Autodesk Inventor part; units mm, degrees
ref_plane "YZ Plane" through (0, 0, 0) normal (1, 0, 0) x (0, 1, 0)
ref_plane "XZ Plane" through (0, 0, 0) normal (0, 1, 0) x (-1, 0, 0)
ref_plane "XY Plane" through (0, 0, 0) normal (0, 0, 1) x (1, 0, 0)
ref_plane "Work Plane1" through (0, 0, 0) normal (0, 0, 1) x (1, 0, 0)
sketch "Sketch1" plane through (0, 0, 0) normal (0, 0, 1) x (1, 0, 0)
  line L0 (0, 75.8) -> (40.7, 75.8)
  line L1 (40.7, 65.2) -> (40.7, 75.8) construction
  line L2 (40.7, 65.2) -> (0, 65.2)
  line L3 (0, 65.2) -> (0, 75.8)
  line L4 (0, 0) -> (0, 65.2) construction
  line L5 (40.7, 0) -> (0, 0)
  line L6 (40.7, 0) -> (40.7, 65.2) construction
  line L7 (0, 65.2) -> (40.7, 65.2)
  line L8 (0, -10.6) -> (40.7, -10.6)
  line L9 (0, 0) -> (0, -10.6)
  line L10 (40.7, -10.6) -> (40.7, 0) construction
  line L11 (40.7, 32.6) -> (0, 32.6) construction
  line L12 (0, 32.6) -> (-300, 32.6) construction
  line L13 (30, 75.8) -> (30, 85.8)
  line L14 (-300, 125.8) -> (-300, 32.6)
  line L15 (-300, -60.6) -> (-300, 32.6)
  line L16 (30, 0) -> (30, 65.2)
  line L17 (-3, 85.8) -> (-3, 95.8)
  line L18 (30, 85.8) -> (-3, 85.8)
  line L19 (-3, 95.8) -> (-300, 125.8)
  line L20 (30, -10.6) -> (30, -20.6)
  line L21 (-3, -20.6) -> (-3, -30.6)
  line L22 (30, -20.6) -> (-3, -20.6)
  line L23 (-3, -30.6) -> (-300, -60.6)
  line L24 (-300, 110.2667) -> (-303, 110.2667)
  line L25 (-303, 110.2667) -> (-303, 79.2)
  line L26 (-303, 79.2) -> (-300, 79.2)
  line L27 (-300, 48.1333) -> (-303, 48.1333)
  line L28 (-303, 48.1333) -> (-303, 32.6)
  line L29 (-303, 32.6) -> (-300, 32.6) construction
  line L30 (-303, 79.2) -> (-303, 48.1333) construction
  line L31 (-303, 110.2667) -> (-303, 125.8) construction
  line L32 (-303, 125.8) -> (-300, 125.8) construction
  line L33 (-301.5, 110.2667) -> (-301.5, 94.7333) construction
  line L34 (-301.5, 94.7333) -> (-303, 94.7333) construction
  line L35 (-300, -45.0667) -> (-303, -45.0667)
  line L36 (-303, -45.0667) -> (-303, -14)
  line L37 (-303, -14) -> (-300, -14)
  line L38 (-300, 17.0667) -> (-303, 17.0667)
  line L39 (-303, 17.0667) -> (-303, 32.6)
  line L40 (-3, 75.8) -> (-3, 85.8)
  dimension "d0" = 300
  dimension "d1" = 10
  dimension "d2" = 50
  dimension "d3" = 30
  dimension "d6" = 10
  dimension "d10" = 3
extrude "Extrusion1" add sketch "Sketch1" along normal blind 3
sketch "Sketch3" plane through (0, 0, 3) normal (0, 0, 1) x (1, 0, 0)
  line L0 (0, 75.8) -> (30, 75.8)
  line L1 (30, 75.8) -> (30, 85.8)
  line L2 (30, 85.8) -> (-3, 85.8)
  line L3 (-3, 85.8) -> (-3, 95.8)
  line L4 (-3, 95.8) -> (-300, 125.8)
  line L5 (-300, 125.8) -> (-300, 110.2667)
  line L6 (-300, 110.2667) -> (-303, 110.2667)
  line L7 (-303, 110.2667) -> (-303, 79.2)
  line L8 (-303, 79.2) -> (-300, 79.2)
  line L9 (-300, 79.2) -> (-300, 48.1333)
  line L10 (-300, 48.1333) -> (-303, 48.1333)
  line L11 (-303, 48.1333) -> (-303, 17.0667)
  line L12 (-303, 17.0667) -> (-300, 17.0667)
  line L13 (-300, 17.0667) -> (-300, -14)
  line L14 (-300, -14) -> (-303, -14)
  line L15 (-303, -14) -> (-303, -45.0667)
  line L16 (-303, -45.0667) -> (-300, -45.0667)
  line L17 (-300, -45.0667) -> (-300, -60.6)
  line L18 (-300, -60.6) -> (-3, -30.6)
  line L19 (-3, -30.6) -> (-3, -20.6)
  line L20 (-3, -20.6) -> (30, -20.6)
  line L21 (30, -20.6) -> (30, -10.6)
  line L22 (30, -10.6) -> (0, -10.6)
  line L23 (0, -10.6) -> (0, 0)
  line L24 (0, 0) -> (30, 0)
  line L25 (30, 0) -> (30, 65.2)
  line L26 (30, 65.2) -> (0, 65.2)
  line L27 (0, 65.2) -> (0, 75.8)
properties part number "Stand 1" material "Wood (Oak)"
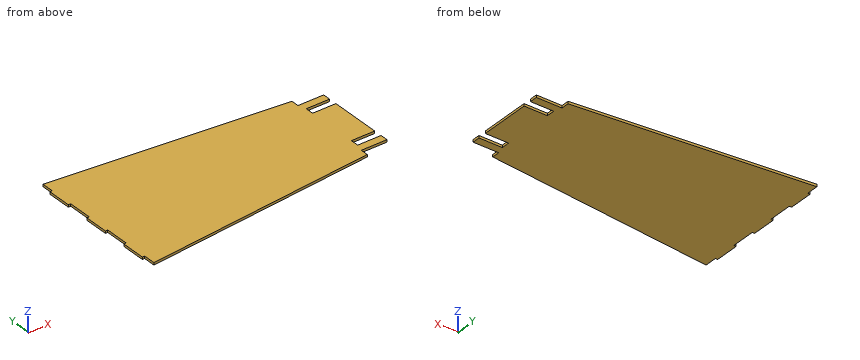
Here's how the part is built. I have some questions about the finished solid (model axes, mm). Round coordinates to 2 decimals unless told otherwise and drop trailing zeros. Loops run counter-clockwise (first coordinate to the right, second up) from the corner with the lowest first, then second, coordinate; pieces in that order, holes last. Notation, with made-up numbers: M -18,30 L 4,30 A22 cw 4,64 Z; hole C 85.5,-31 d3. An arc over 180 degrees is marked long. Write each question's results on one line, items separated by ' | '. Start each with the question number.
(1) I want a section at D-D (x = -39). Please give me the cut outline in (y, z), then the cut area to 3 significant figures.
(2) I want a section at B-B (z = 2). Please give me the cut outline in (x, y), then the cut area to 3 significant figures.
(3) I want a section at A-A (x = 7). Please give me the cut outline in (y, z).
(4) Will these pins go through, and if not, where does the flat tip stop? P1, Ø0.9, axis at x = 9, z = 1.5, coming from the +Y side; P2, Ø0.9, axis at y = -5.5, z = 2, coming from the +X side; P3, Ø0.9, axis at y = -56, z = 1.5, coming from the -X side.
(5) I want a section at C-C (y = 107). Please give me the cut outline in (x, z).
(6) If I drill on probe 1 along Y at (x, z) = (2, 1.2); probe 2 along X at (y, z) = (9, 0.65); probe 3 along X at (y, z) = (68, 0.1), over which ranges is the centre line in solid material (lowest first)? Write a range as from..to.
Solved:
1) outline: M -34.24,0 L 99.44,0 L 99.44,3 L -34.24,3 Z | area: 401 mm²
2) outline: M -303,-45.07 L -300,-45.07 L -300,-60.6 L -3,-30.6 L -3,-20.6 L 30,-20.6 L 30,-10.6 L 0,-10.6 L 0,0 L 30,0 L 30,65.2 L 0,65.2 L 0,75.8 L 30,75.8 L 30,85.8 L -3,85.8 L -3,95.8 L -300,125.8 L -300,110.27 L -303,110.27 L -303,79.2 L -300,79.2 L -300,48.13 L -303,48.13 L -303,17.07 L -300,17.07 L -300,-14 L -303,-14 Z | area: 49,600 mm²
3) outline: M -20.6,0 L -10.6,0 L -10.6,3 L -20.6,3 Z; M 0,0 L 65.2,0 L 65.2,3 L 0,3 Z; M 75.8,0 L 85.8,0 L 85.8,3 L 75.8,3 Z
4) P1: stops at y = 85.8 | P2: stops at x = 0 | P3: stops at x = -300
5) outline: M -303,0 L -113.88,0 L -113.88,3 L -303,3 Z
6) probe 1: y = -20.6..-10.6, 0..65.2, 75.8..85.8 | probe 2: x = -300..30 | probe 3: x = -300..0
